Source: CAD feature listing. Evaluate the final solid. Frame: model axes, mm. Face numbers are marked on the shaded views. Give positions to 0.01 mm unless a question says otherwise; leave off trailing zeros. Write each loop counter-clockwise with the first axis right and the second up, starting at its lowest first coordinate (ties: lowest second). Pieces come first, ordered by that corner, then holes.
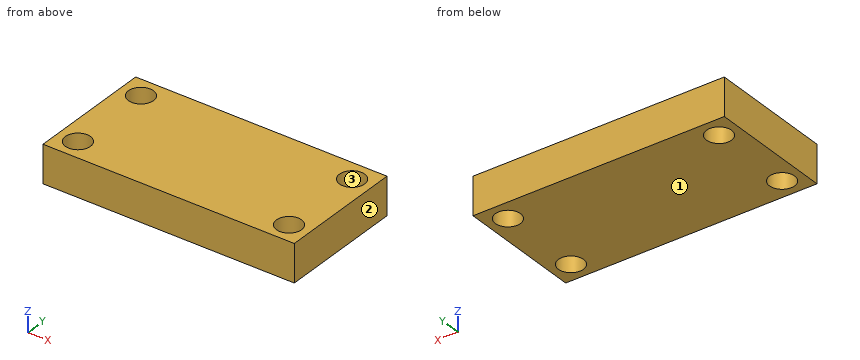
```python
from build123d import *

# Parameters (mm, degrees)
SKETCH001_W  = 100
SKETCH001_H  = 50
SKETCH001_R  = 5
PAD_DEPTH    = 15
PAD001_DEPTH = 15


with BuildPart() as part:
    # Sketch001 → Pad (new body)
    with BuildSketch(Plane.XY):
        with Locations((50, 25)):
            Rectangle(SKETCH001_W, SKETCH001_H)
        with Locations((92, 42)):
            Circle(SKETCH001_R, mode=Mode.SUBTRACT)
        with Locations((8, 42)):
            Circle(SKETCH001_R, mode=Mode.SUBTRACT)
        with Locations((92, 8)):
            Circle(SKETCH001_R, mode=Mode.SUBTRACT)
        with Locations((8, 8)):
            Circle(SKETCH001_R, mode=Mode.SUBTRACT)
    extrude(amount=PAD_DEPTH)

    # Sketch001 → Pad001 (join)
    with BuildSketch(Plane.XY):
        with Locations((50, 25)):
            Rectangle(SKETCH001_W, SKETCH001_H)
        with Locations((92, 42)):
            Circle(SKETCH001_R, mode=Mode.SUBTRACT)
        with Locations((8, 42)):
            Circle(SKETCH001_R, mode=Mode.SUBTRACT)
        with Locations((92, 8)):
            Circle(SKETCH001_R, mode=Mode.SUBTRACT)
        with Locations((8, 8)):
            Circle(SKETCH001_R, mode=Mode.SUBTRACT)
    extrude(amount=PAD001_DEPTH)


solid = part.part
```
1. Cut plane A-A, the plane y = 8. Return the cut outline in (x, z).
2. Line query: L1, parallel to Y at x = 92, z = 7.25; L2, parallel to X at y = 11, z = 13; L3, parallel to X at y = 45.5, z = 10.75. Output: solid intervals per line, ascending.
3. Cut plane C-C, the plane z = 9.75. Return the cut outline in (x, y).
4. Cut plane B-B, the plane x = 92. Return the cut outline in (y, z), then the cut area to 3 significant figures.
5. Contact query for a flat-ended pin moving along its axis: P1, Ø8, axis at x = 8, y = 8, coming from the +Z side. Output: stop coordinate, or through.
6. Mould query, pull axis X, two halves, no side actions, for the marked faces 1, 2 and 3. Classes: +X half, -X half, draft (parallel to the pull), parting line (faces both ways), or undercut.
Response values:
1. outline: (0, 0) - (3, 0) - (3, 15) - (0, 15) - close; (13, 0) - (87, 0) - (87, 15) - (13, 15) - close; (97, 0) - (100, 0) - (100, 15) - (97, 15) - close
2. L1: y = 0 to 3, 13 to 37, 47 to 50
2. L2: x = 0 to 4, 12 to 88, 96 to 100
2. L3: x = 0 to 4.43, 11.57 to 88.43, 95.57 to 100
3. outline: (0, 0) - (100, 0) - (100, 50) - (0, 50) - close; hole circle Ø10 at (8, 8); hole circle Ø10 at (8, 42); hole circle Ø10 at (92, 8); hole circle Ø10 at (92, 42)
4. outline: (0, 0) - (3, 0) - (3, 15) - (0, 15) - close; (13, 0) - (37, 0) - (37, 15) - (13, 15) - close; (47, 0) - (50, 0) - (50, 15) - (47, 15) - close
4. area: 450 mm2
5. P1: passes through
6. face 1: draft
6. face 2: +X half
6. face 3: undercut
